Autodesk Inventor part; units mm, degrees
ref_plane "YZ Plane" through (0, 0, 0) normal (1, 0, 0) x (0, 1, 0)
ref_plane "XZ Plane" through (0, 0, 0) normal (0, 1, 0) x (-1, 0, 0)
ref_plane "XY Plane" through (0, 0, 0) normal (0, 0, 1) x (1, 0, 0)
sketch "Sketch1" plane through (0, 0, 0) normal (0, 0, 1) x (1, 0, 0)
  arc A0 (-6.1315, 4.735) -> (6.1315, 4.735) centre (0, 0) ccw
  line L0 (0, 0) -> (13.0157, 0) construction
  line L1 (7.747, 4.735) -> (7.747, 11.466)
  line L2 (7.747, 11.466) -> (-7.747, 11.466)
  line L3 (-7.747, 11.466) -> (-7.747, 4.735)
  line L4 (-7.747, 4.735) -> (-6.1315, 4.735)
  line L5 (6.1315, 4.735) -> (7.747, 4.735)
  dimension "d0" = 15.494
  dimension "d1" = 6.731
  dimension "d2" = 15.494
  dimension "d3" = 7.747
extrude "Extrusion1" add sketch "Sketch1" along normal blind 1.143
sketch "Sketch2" plane through (0, 0, 1.143) normal (0, 0, 1) x (1, 0, 0)
  line L0 (7.747, 11.466) -> (-7.747, 11.466)
  point P0 (-7.747, 4.735)
  point P1 (-5, 8.1005)
  point P2 (0, 8.1005)
  point P3 (5, 8.1005)
  dimension "d6" = 5
  dimension "d7" = 5
  dimension "d8" = 6.731
  dimension "d9" = 3.3655
hole "Hole1" at (-5, 8.1005, 1.143) at (0, 8.1005, 1.143) at (5, 8.1005, 1.143) direction (0, 0, -1) diameter 1.4478 end through all
properties part number "Potenciometro - Base"
Here's how the part is built. I have some questions about the finished solid (model axes, mm). Give positions to 0.01 mm unless a question says otherwise; leave off trailing zeros. Order: outer loops, then holes, each group sorted by start corner. A loop starts at its lowest first (then second) coordinate and runs counter-clockwise, first axis right, second up. Notation, with made-up numbers: (49, 8.5) -> (77, 8.5) arc R24 ccw to (77, 37.5) -> close; hole circle Ø1 at (81.25, 8.25). An arc over 180 degrees is marked (long way). Use a Markdown table: item, result. Add a question column.
Item 1: If we mould it in two halves opening along Y, with no side actions, what happens to faces 1 (the face through (-7, 4.735, 0.6)), 2 (the face through (0.1, 11.466, 0.6)), 3 (the face through (-7.747, 8.1, 0.6))? For each: pulls with the +Y half, pulls with the -Y half, needs draft (parallel to the pull), parting line crosses it, or undercut.
Item 2: Imagine slicing it at D-D on y = 1.75. Please give me the cut outline in (x, z), plus the area to 3 significant figures.
Item 3: Imagine slicing it at B-B on z = 0.8. Please give me the cut outline in (x, y) (1 decimal), plus the area to 3 significant figures.
Item 4: Will these pins go through, and if not, where does the flat tip stop? pin 1 (2 mm diameter, centred on x = 3.5, y = -4, fed in from -Z); pin 2 (0.6 mm diameter, centred on x = 7, z = 0.5, fed in from -Y).
Item 5: I need wall thicknesses on line 1 (Y direction, x = 0, z = 0.45); line 2 (Y direction, x = 0.5, z = 0.9); line 3 (X direction, y = 7.75, z = 0.95). Which ranges of each line are inside material? Lowest first, please.
Item 6: Imagine slicing it at C-C on x = -5. Please give me the cut outline in (y, z), plus the area to 3 significant figures.
Item 7: Imagine slicing it at A-A on x = 0. Please give me the cut outline in (y, z), plus the area to 3 significant figures.
Data:
| question | item | result |
|---|---|---|
| 1 | face 1 | undercut |
| 1 | face 2 | pulls with the +Y half |
| 1 | face 3 | needs draft |
| 2 | outline | (-7.55, 0) -> (7.55, 0) -> (7.55, 1.14) -> (-7.55, 1.14) -> close |
| 2 | area | 17.3 mm² |
| 3 | outline | (-7.7, 4.7) -> (-6.1, 4.7) arc R7.7 ccw (long way) to (6.1, 4.7) -> (7.7, 4.7) -> (7.7, 11.5) -> (-7.7, 11.5) -> close; hole circle Ø1.4 at (-5, 8.1); hole circle Ø1.4 at (0, 8.1); hole circle Ø1.4 at (5, 8.1) |
| 3 | area | 262 mm² |
| 4 | pin 1 | stops at z = 0 |
| 4 | pin 2 | stops at y = -3.89 |
| 5 | line 1 | y = -7.75 to 7.38, 8.82 to 11.47 |
| 5 | line 2 | y = -7.73 to 7.58, 8.62 to 11.47 |
| 5 | line 3 | x = -7.75 to -5.63, -4.37 to -0.63, 0.63 to 4.37, 5.63 to 7.75 |
| 6 | outline | (-5.92, 0) -> (7.38, 0) -> (7.38, 1.14) -> (-5.92, 1.14) -> close; (8.82, 0) -> (11.47, 0) -> (11.47, 1.14) -> (8.82, 1.14) -> close |
| 6 | area | 18.2 mm² |
| 7 | outline | (-7.75, 0) -> (7.38, 0) -> (7.38, 1.14) -> (-7.75, 1.14) -> close; (8.82, 0) -> (11.47, 0) -> (11.47, 1.14) -> (8.82, 1.14) -> close |
| 7 | area | 20.3 mm² |
